Build history of the part. All positions in model axes, mm. A direction names the side the tool comes from. Round coordinates to 2 decimals unless told otherwise and drop trailing zeros. Order: outer loops, then holes, each group sorted by start corner. A loop starts at its lowest first (then second) coordinate and runs counter-clockwise, first axis right, second up. Notation, with made-up numbers: (9.5, 88) -> (16.5, 88) arc R16 ccw to (16.5, 118) -> close; hole circle Ø2 at (42, 20.25). An arc over 180 degrees is marked (long way). Use a Markdown table: item, result. Add a question column.
Item 1: Pin check, flat tips, straight feed: pin 1 (3 mm diameter, centred on x = -29.5, z = 3.5, fed in from -Y); pin 2 (0.8 mm diameter, centred on x = -29.5, z = 4.5, fed in from +Y); pin 3 (1.1 mm diameter, centred on y = -62.5, z = 5.5, fed in from -X). Stop position of each tip, or through.
Item 2: Slice it at C-C, the plane x = -23.5. Give the cut face in (y, z), plus the area to 4 significant figures.
Item 3: Slice it at A-A, the plane x = 12.5. Give the cut face in (y, z), plus the area to 3 significant figures.
Item 4: Slice it at B-B, the plane y = 28. Give the cut face in (x, z), plus the area to 3 significant figures.
Item 5: 3-axis set-ups, long thin cutter, end or side, ignore diameter. For faces 1 (the face through (-30, 12.383, 4)), 2 (the face through (23.747, 56.409, 0.493)), 3 (the face through (0, 1, 0)), 4 (the face through (0, 62.15, 5)): which of +Z, -Z, +X, -X, +Y, -Y reach the whole face in a straight line?
Item 6: Slice it at D-D, the plane y = 9. Give the cut face in (x, z), plus the area to 3 significant figures.
Item 7: Two-plate mould, pull along X, no slides. Class faces 5 (the face through (29.55, -1, 5)), 6 (the face through (-30, 0, 10.1)), 7 (the face through (28.87, -61.55, 4.98)), 8 (the face through (-28.87, 61.55, 4.98)): released by +X, released by -X, zero draft, split by the parting line, or undercut.
Item 8: Probe L1, parallel to Y at x = -22, z = 9; L2, parallel to X at y = -29.5, z = 3; L3, parallel to Z at x = 18, y = 11.5. List the from-to ranges inside material, lowest first.
from build123d import *

# Parameters (mm, degrees)
F1_DEPTH = 10.1
F2_T     = -1
F4_DEPTH = 25
F5_W     = 45.166726
F5_H     = 8.800845
F6_DEPTH = 2.5
F8_DEPTH = 2.5


with BuildPart() as f1:
    # F0 (on Top) → F1 (new body)
    with BuildSketch(Plane.XY):
        with BuildLine():
            Line((24.95, 63.15), (-24.95, 63.15))
            ThreePointArc((-24.95, 63.15), (-28.909798, 61.509798), (-30.55, 57.55))
            Line((-30.55, 57.55), (-30.55, -57.55))
            ThreePointArc((-30.55, -57.55), (-28.909798, -61.509798), (-24.95, -63.15))
            Line((-24.95, -63.15), (24.95, -63.15))
            ThreePointArc((24.95, -63.15), (28.909798, -61.509798), (30.55, -57.55))
            Line((30.55, -57.55), (30.55, 57.55))
            ThreePointArc((30.55, 57.55), (28.909798, 61.509798), (24.95, 63.15))
        make_face()
    extrude(amount=F1_DEPTH)

    # F2
    f2_openings = [f1.faces().sort_by_distance(p)[0] for p in [
        (0, 0, 10.1),
    ]]
    offset(amount=F2_T, openings=f2_openings)

    # F3 (on face) → F4 (cut)
    with BuildSketch(Plane(origin=(0, 0, 0), x_dir=(1, 0, 0), z_dir=(0, 0, -1))):
        with BuildLine():
            Line((0.899941, -57.55), (20.95, -57.55))
            ThreePointArc((20.95, -57.55), (23.778427, -56.378427), (24.95, -53.55))
            Line((24.95, -53.55), (24.95, -46.00715))
            ThreePointArc((24.95, -46.00715), (24.832843, -45.724307), (24.55, -45.60715))
            Line((24.55, -45.60715), (6.199941, -45.60715))
            ThreePointArc((6.199941, -45.60715), (2.452275, -47.159484), (0.899941, -50.90715))
            Line((0.899941, -50.90715), (0.899941, -57.55))
        make_face()
    extrude(amount=-F4_DEPTH, mode=Mode.SUBTRACT)

    # F5 (on face) → F6 (cut)
    with BuildSketch(Plane(origin=(-30.55, 0, 0), x_dir=(0, -1, 0), z_dir=(-1, 0, 0))):
        with Locations((-34.966637, 4.400422)):
            Rectangle(F5_W, F5_H)
    extrude(amount=-F6_DEPTH, mode=Mode.SUBTRACT)

    # F7 (on face) → F8 (cut)
    with BuildSketch(Plane.XZ.offset(63.15)):
        with BuildLine():
            Line((5.738557, 7.637859), (-5.738557, 7.637859))
            ThreePointArc((-5.738557, 7.637859), (-6.975994, 7.125296), (-7.488557, 5.887859))
            Line((-7.488557, 5.887859), (-7.488557, 4.212141))
            ThreePointArc((-7.488557, 4.212141), (-6.975994, 2.974704), (-5.738557, 2.462141))
            Line((-5.738557, 2.462141), (5.738557, 2.462141))
            ThreePointArc((5.738557, 2.462141), (6.975994, 2.974704), (7.488557, 4.212141))
            Line((7.488557, 4.212141), (7.488557, 5.887859))
            ThreePointArc((7.488557, 5.887859), (6.975994, 7.125296), (5.738557, 7.637859))
        make_face()
    extrude(amount=-F8_DEPTH, mode=Mode.SUBTRACT)


solid = f1.part
Check sheet entries:
| question | item | result |
|---|---|---|
| 1 | pin 1 | y = -62.25 |
| 1 | pin 2 | y = 61.31 |
| 1 | pin 3 | x = -28.41 |
| 2 | outline | (-63.15, 0) -> (63.15, 0) -> (63.15, 10.1) -> (62.15, 10.1) -> (62.15, 1) -> (-62.15, 1) -> (-62.15, 10.1) -> (-63.15, 10.1) -> close |
| 2 | area | 144.5 mm2 |
| 3 | outline | (-63.15, 0) -> (45.61, 0) -> (45.61, 1) -> (-62.15, 1) -> (-62.15, 10.1) -> (-63.15, 10.1) -> close; (57.55, 0) -> (63.15, 0) -> (63.15, 10.1) -> (62.15, 10.1) -> (62.15, 1) -> (57.55, 1) -> close |
| 3 | area | 133 mm2 |
| 4 | outline | (-30.55, 8.8) -> (-29.55, 8.8) -> (-29.55, 10.1) -> (-30.55, 10.1) -> close; (-28.05, 0) -> (30.55, 0) -> (30.55, 10.1) -> (29.55, 10.1) -> (29.55, 1) -> (-28.05, 1) -> close |
| 4 | area | 69.0 mm2 |
| 5 | face 1 | -Z, -X |
| 5 | face 2 | +Z, -Z |
| 5 | face 3 | -Z, +X, -X, +Y, -Y |
| 5 | face 4 | +Z |
| 6 | outline | (-30.55, 0) -> (30.55, 0) -> (30.55, 10.1) -> (29.55, 10.1) -> (29.55, 1) -> (-29.55, 1) -> (-29.55, 10.1) -> (-30.55, 10.1) -> close |
| 6 | area | 79.3 mm2 |
| 7 | face 5 | undercut |
| 7 | face 6 | zero draft |
| 7 | face 7 | released by +X |
| 7 | face 8 | released by -X |
| 8 | L1 | -63.15 to -62.15, 62.15 to 63.15 |
| 8 | L2 | -30.55 to -29.55, 29.55 to 30.55 |
| 8 | L3 | 0 to 1 |
